from build123d import *

# Parameters (mm, degrees)
SKETCH1_R               = 5.25
SKETCH1_R_2             = 3.9
SKETCH1_W               = 20.5
SKETCH1_H               = 20.7
BOSS_EXTRUDE1_DEPTH     = 4
SKETCH2_R               = 5.25
BOSS_EXTRUDE2_DEPTH     = 11
SKETCH3_W               = 20.5
SKETCH3_H               = 20.7
BOSS_EXTRUDE3_DEPTH     = 17
BOSS_EXTRUDE4_DEPTH     = 4
BOSS_EXTRUDE6_DEPTH     = 4
FILLET8_R               = 2
SKETCH7_R               = 2.6
CUT_EXTRUDE1_DEPTH      = 6
SKETCH9_R               = 3
CUT_EXTRUDE2_DEPTH      = 25.5
CUT_EXTRUDE2_DEPTH_BACK = 15.75
SKETCH10_R              = 3.9
BOSS_EXTRUDE7_DEPTH     = 8


with BuildPart() as part:
    # Sketch1 → Boss-Extrude1 (new body)
    with BuildSketch(Plane.XY):
        with BuildLine():
            Line((-29.25, -25.65), (-29.25, -54.35))
            Line((-29.25, -54.35), (-20.75, -70))
            Line((-20.75, -70), (-0.75, -70))
            Line((-0.75, -70), (-0.75, -32.65))
            Line((-0.75, -32.65), (9.446850202, -3.279789821))
            ThreePointArc((9.446850202, -3.279789821), (8.962582875, 4.435325039), (3.122498999, 9.5))
            Line((3.122498999, 9.5), (-3.122498999, 9.5))
            ThreePointArc((-3.122498999, 9.5), (-6.041680661, 7.968569181), (-8.304318811, 5.571201763))
            Line((-8.304318811, 5.571201763), (-29.25, -25.65))
        make_face()
        Circle(SKETCH1_R, mode=Mode.SUBTRACT)
        with Locations((-11, -21.5)):
            Circle(SKETCH1_R_2, mode=Mode.SUBTRACT)
        with Locations((-15, -40)):
            Rectangle(SKETCH1_W, SKETCH1_H, mode=Mode.SUBTRACT)
    extrude(amount=BOSS_EXTRUDE1_DEPTH)

    # Sketch2 → Boss-Extrude2 (add)
    with BuildSketch(Plane.XY.offset(4)):
        with BuildLine():
            Line((3.122498999, 9.5), (-3.122498999, 9.5))
            ThreePointArc((-3.122498999, 9.5), (0, -10), (3.122498999, 9.5))
        make_face()
        Circle(SKETCH2_R, mode=Mode.SUBTRACT)
    extrude(amount=BOSS_EXTRUDE2_DEPTH)

    # Sketch3 → Boss-Extrude3 (add)
    with BuildSketch(Plane.XY.offset(4)):
        Polygon((-29.25, -25.65), (-29.25, -54.35), (-20.75, -70), (-0.75, -70), (-0.75, -25.65), align=None)
        with Locations((-15, -40)):
            Rectangle(SKETCH3_W, SKETCH3_H, mode=Mode.SUBTRACT)
        with BuildLine():
            Line((-6.75, -54.35), (-21.33587702, -54.35))
            ThreePointArc((-21.33587702, -54.35), (-23.054759053, -55.327530168), (-23.093382043, -57.304555444))
            Line((-23.093382043, -57.304555444), (-18.938429966, -64.954555444))
            ThreePointArc((-18.938429966, -64.954555444), (-18.203394775, -65.718882033), (-17.180924944, -66))
            Line((-17.180924944, -66), (-6.75, -66))
            ThreePointArc((-6.75, -66), (-5.335786438, -65.414213562), (-4.75, -64))
            Line((-4.75, -64), (-4.75, -56.35))
            ThreePointArc((-4.75, -56.35), (-5.335786438, -54.935786438), (-6.75, -54.35))
        make_face(mode=Mode.SUBTRACT)
    extrude(amount=BOSS_EXTRUDE3_DEPTH)

    # Sketch4 → Boss-Extrude4 (add)
    with BuildSketch(Plane(origin=(-8.304318811, 5.571201763, 0), x_dir=(0, 0, 1), z_dir=(-0.830431881, 0.557120176, 0))):
        Polygon((4, -37.596342907), (21, -37.596342907), (21, -32.596342907), (12, 0), (4, 0), align=None)
    extrude(amount=-BOSS_EXTRUDE4_DEPTH)

    # Sketch6 → Boss-Extrude6 (add)
    with BuildSketch(Plane(origin=(9.446850202, -3.279789821, 0), x_dir=(0, 0, -1), z_dir=(0.94468502, -0.327978982, 0))):
        Polygon((-4, -31.089950145), (-21, -31.089950145), (-21, -23.089950145), (-10, 0), (-4, 0), align=None)
    extrude(amount=-BOSS_EXTRUDE6_DEPTH)

    # Fillet8
    fillet8_edges = [part.edges().sort_by_distance(p)[0] for p in [
        (-24.433229244, -25.65, 12.5),
        (-2.553931563, -25.65, 12.5),
        (3.044278264, -9.525354054, 8.905590949),
        (-9.439552697, -3.300733991, 9.104418373),
        (-0.75, -32.65, 10.5),
    ]]
    fillet(fillet8_edges, radius=FILLET8_R)

    # Sketch7 → Cut-Extrude1 (cut)
    with BuildSketch(Plane(origin=(0, 9.5, 0), x_dir=(1, 0, 0), z_dir=(0, 1, 0))):
        with Locations(Location((0, -7.5, 0), (0, 0, 270))):  # turned: the seam where the file's is
            Circle(SKETCH7_R)
    extrude(amount=-CUT_EXTRUDE1_DEPTH, mode=Mode.SUBTRACT)

    # Sketch9 → Cut-Extrude2 (cut, two sides)
    with BuildSketch(Plane.ZY.offset(4.75)) as cut_extrude2_sk:
        with Locations(Location((10.5, -40, 0), (0, 0, 270))):  # turned: the seam where the file's is
            Circle(SKETCH9_R)
    extrude(amount=CUT_EXTRUDE2_DEPTH, mode=Mode.SUBTRACT)
    extrude(cut_extrude2_sk.sketch, amount=-CUT_EXTRUDE2_DEPTH_BACK, mode=Mode.SUBTRACT)

    # Sketch10 → Boss-Extrude7 (add)
    with BuildSketch(Plane.XY.offset(4)):
        with BuildLine():
            Line((-11.28568656, -6.052543173), (-22.343947541, -22.535759647))
            ThreePointArc((-22.343947541, -22.535759647), (-22.44780482, -24.591148048), (-20.683083779, -25.65))
            Line((-20.683083779, -25.65), (-3.976672485, -25.65))
            ThreePointArc((-3.976672485, -25.65), (-2.817344215, -25.279711006), (-2.087302444, -24.305957964))
            Line((-2.087302444, -24.305957964), (1.957451524, -12.655764834))
            ThreePointArc((1.957451524, -12.655764834), (1.69449722, -10.835860199), (0.05673457, -9.999839058))
            ThreePointArc((0.05673457, -9.999839058), (-4.462214417, -8.949225805), (-8.020685665, -5.972319605))
            ThreePointArc((-8.020685665, -5.972319605), (-9.6739495, -5.167386975), (-11.28568656, -6.052543173))
        make_face()
        with Locations((-11, -21.5)):
            Circle(SKETCH10_R, mode=Mode.SUBTRACT)
    extrude(amount=BOSS_EXTRUDE7_DEPTH)


solid = part.part
Here's how the part is built. I have some questions about the finished solid (model axes, mm). A direction names the side the tool comes from. Round coordinates to 2 decimals unless told otherwise and drop trailing zeros. Write each loop counter-clockwise with the first axis right and the second up, starting at its lowest first coordinate (ties: lowest second). Pieces come first, ordered by that corner, then holes.
1. Will these pins go through, and if not, where does the flat tip stop? pin 1 Ø9 at (x, y) = (-11, -21.5) entering from -Z; pin 2 Ø8 at (y, z) = (-49, 17.5) entering from +X; pin 3 Ø8.5 at (x, z) = (-13, 16) entering from +Y; pin 4 Ø4 at (y, z) = (-22, 12.5) entering from +X.
2. I need wall thicknesses on L1, parallel to X at y = -30.5, z = 16.75; L2, parallel to X at y = -40.5, z = 14.75; L3, parallel to Z at x = -2, y = -40. Which ranges of each line are inside material? Lowest first, please.
3. Suppose I cut it at B-B (z = 2.25). List the corners of the cut face in (x, y) for me, and give its area (3 significant figures).
4. Suppose I cut it at D-D (z = 19.25). List the corners of the cut face in (x, y) for me, and give its area (3 significant figures).
5. For faces 1 (the flat face through (-25.25, -38, 8)), 2 (the cylindrical face through (-2.803, -25.27, 16.437)), 3 (the flat face through (-25.06, -62.065, 10.353)), which set-ups out of +Z, -Z, +X, -X, +Y, -Y let a thin tool reach every point of the face, with its end or its side?
6. Suppose I cut it at A-A (y = -40). List the corners of the cut face in (x, z) for me, and give its area (3 significant figures).
7. If we mould it in two halves opening along Z, with no side actions, what happens to faces 4 (the cylindrical face through (-5.35, -65.43, 12.38)), 5 (the flat face through (-1, -30, 0)), 6 (the flat face through (-14, -51, 21)), 7 (the cylindrical face through (-2.8, -37, 10.6))? For each: released by +Z, released by -Z, zero draft, split by the parting line, or undercut.
8. Suppose I cut it at C-C (x = -12.5). List the corners of the cut face in (y, z) for me, and give its area (3 significant figures).
Answer sheet:
1. pin 1: stops at z = 0
1. pin 2: stops at x = -0.75
1. pin 3: stops at y = 4.62
1. pin 4: stops at x = 3.64
2. L1: x = -29.25 to -25.25, -4.75 to 0
2. L2: x = -29.25 to -25.25, -4.75 to -0.75
2. L3: z = 0 to 7.5, 13.5 to 21
3. outline: (-29.25, -54.35) - (-20.75, -70) - (-0.75, -70) - (-0.75, -32.99) arc R2 cw to (-0.64, -32.33) - (9.45, -3.28) arc R10 ccw to (3.12, 9.5) - (-3.12, 9.5) arc R10 ccw to (-8.3, 5.57) - (-29.25, -25.65) - close; hole (-25.25, -50.35) - (-4.75, -50.35) - (-4.75, -29.65) - (-25.25, -29.65) - close; hole circle Ø7.8 at (-11, -21.5); hole circle Ø10.5 at (0, 0)
3. area: 1,490 mm2
4. outline: (-29.25, -54.35) - (-20.75, -70) - (-0.75, -70) - (-0.75, -32.99) arc R2 cw to (-0.64, -32.33) - (3.08, -21.62) - (-0.7, -20.31) - (-2.09, -24.31) arc R2 cw to (-3.98, -25.65) - (-20.68, -25.65) arc R2 cw to (-22.34, -22.54) - (-19.61, -18.46) - (-22.93, -16.23) - (-29.25, -25.65) - close; hole (-25.25, -50.35) - (-4.75, -50.35) - (-4.75, -29.65) - (-25.25, -29.65) - close; hole (-23.09, -57.3) - (-18.94, -64.95) arc R2 ccw to (-17.18, -66) - (-6.75, -66) arc R2 ccw to (-4.75, -64) - (-4.75, -56.35) arc R2 ccw to (-6.75, -54.35) - (-21.34, -54.35) arc R2 ccw to start
4. area: 654 mm2
5. face 1: +Z, -Z
5. face 2: +Z
5. face 3: +Z, -Z, -X, -Y
6. outline: (-29.25, 0) - (-25.25, 0) - (-25.25, 7.5) - (-29.25, 7.5) - close; (-29.25, 13.5) - (-25.25, 13.5) - (-25.25, 21) - (-29.25, 21) - close; (-4.75, 0) - (-0.75, 0) - (-0.75, 7.5) - (-4.75, 7.5) - close; (-4.75, 13.5) - (-0.75, 13.5) - (-0.75, 21) - (-4.75, 21) - close
6. area: 120 mm2
7. face 4: zero draft
7. face 5: released by -Z
7. face 6: released by +Z
7. face 7: undercut
8. outline: (-70, 0) - (-50.35, 0) - (-50.35, 21) - (-54.35, 21) - (-54.35, 4) - (-66, 4) - (-66, 21) - (-70, 21) - close; (-29.65, 0) - (-25.1, 0) - (-25.1, 12) - (-25.65, 12) - (-25.65, 21) - (-29.65, 21) - close; (-17.9, 0) - (-0.68, 0) - (-0.68, 14.08) - (-7.86, 15.73) - (-7.86, 12) - (-17.9, 12) - close
8. area: 533 mm2
